Geometry: see drawing. Coordinates: mm, zero at the bounding-box minimum. Coordinates: 2 decimals unless noted, no trailing zeros. Write each loop counter-clockwise with the first axis right and the second up, starting at its lowest first coordinate (ties: lowest second). Pieces come first, ordered by that corner, then holes.
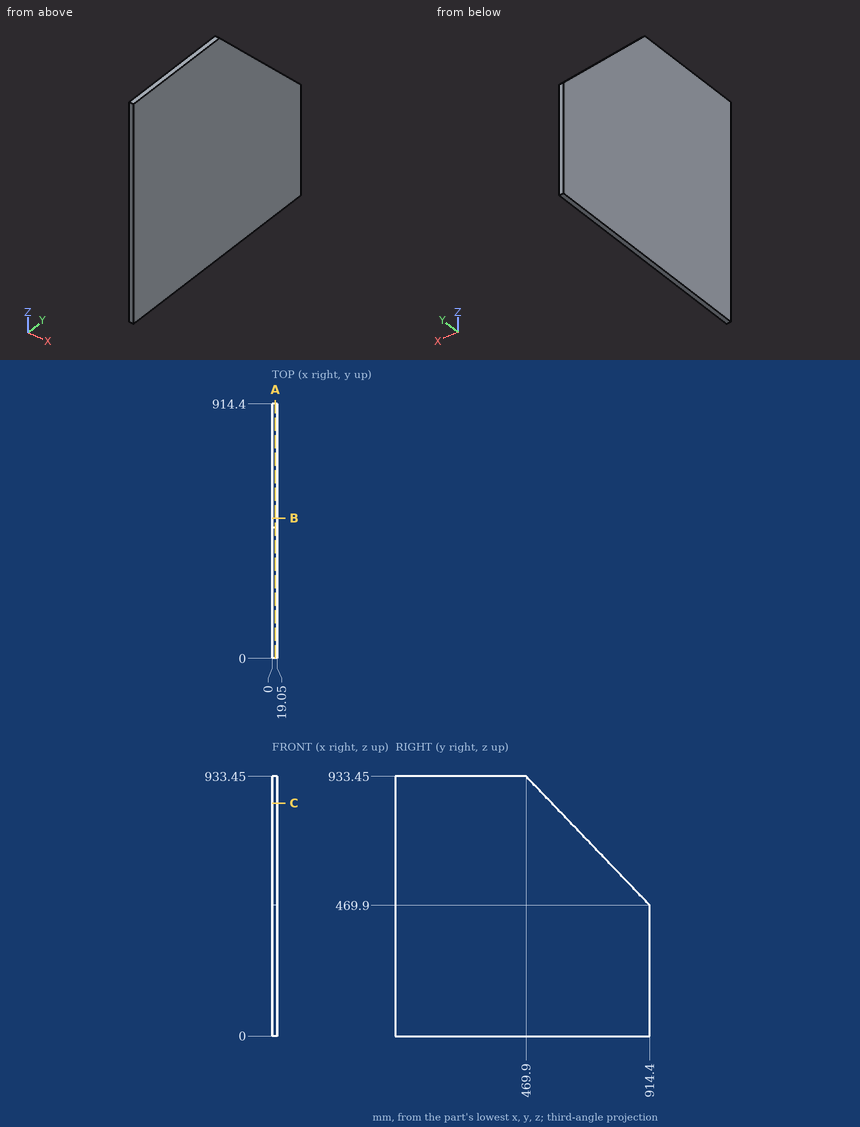
Item 1: Section B-B, the plane y = 504.5. Output: boundary loops of the cut face in (x, z).
Derived:
outline: (0, 0) - (19.05, 0) - (19.05, 897.37) - (0, 897.37) - close
Item 2: Pin query (flat end, axial travel): pin 1 (5 mm diameter, centred on x = 9, z = 563.5, fed in from +Y); pin 2 (2 mm diameter, centred on x = 8.5, y = 626, fed in from +Z). Return the tip coordinate at first contact, or that it passes through.
Derived:
pin 1: stops at y = 827.04
pin 2: stops at z = 771.7
Item 3: Section A-A, the plane x = 11.25. Output: boundary loops of the cut face in (y, z).
Derived:
outline: (0, 0) - (914.4, 0) - (914.4, 469.9) - (469.9, 933.45) - (0, 933.45) - close
Item 4: Section C-C, the plane z = 837.5. Output: boundary loops of the cut face in (x, y).
Derived:
outline: (0, 0) - (19.05, 0) - (19.05, 561.91) - (0, 561.91) - close
Item 5: Material intervals for probe 1 along Z at (x, y) = (1, 567); probe 2 along Z at (x, y) = (4.5, 711); probe 3 along Y at (x, z) = (7.5, 848.5), sorted ascending.
Derived:
probe 1: z = 0 to 832.19
probe 2: z = 0 to 682.02
probe 3: y = 0 to 551.36
